from build123d import *

# Parameters (mm, degrees)
BOSS_EXTRUDE1_DEPTH      = 40
BOSS_EXTRUDE1_DEPTH_BACK = 24.13
SKETCH1_W                = 138
SKETCH1_H                = 88
SHELL1_T                 = -4
SKETCH10_W               = 12.954
SKETCH10_H               = 10.922
CUT_EXTRUDE1_DEPTH       = 4
SKETCH12_W               = 9.254
SKETCH12_H               = 11.254
CUT_EXTRUDE2_DEPTH       = 4


with BuildPart() as part:
    # Sketch1 → Boss-Extrude1 (new, two sides: drawn at the far end of the back side and taken through both)
    with BuildSketch(Plane(origin=(0, 0, 0), x_dir=(1, 0, 0), z_dir=(0, 1, 0)).offset(-BOSS_EXTRUDE1_DEPTH_BACK)):
        with Locations((29.3125, -12.885)):
            Rectangle(SKETCH1_W, SKETCH1_H)
    extrude(amount=BOSS_EXTRUDE1_DEPTH + BOSS_EXTRUDE1_DEPTH_BACK)

    # Shell1
    shell1_openings = [part.faces().sort_by_distance(p)[0] for p in [
        (29.3125, 40, 12.885),
    ]]
    offset(amount=SHELL1_T, openings=shell1_openings, kind=Kind.INTERSECTION)

    # Sketch10 → Cut-Extrude1 (cut)
    with BuildSketch(Plane.ZY.offset(-98.3125)):
        with Locations((-10.795, -11.176)):
            Rectangle(SKETCH10_W, SKETCH10_H)
    extrude(amount=CUT_EXTRUDE1_DEPTH, mode=Mode.SUBTRACT)

    # Sketch12 → Cut-Extrude2 (cut)
    with BuildSketch(Plane.ZY.offset(-98.3125)):
        with Locations((18.36, -11.01)):
            Rectangle(SKETCH12_W, SKETCH12_H)
    extrude(amount=CUT_EXTRUDE2_DEPTH, mode=Mode.SUBTRACT)


solid = part.part
The listing builds one solid part. Answer for the finished solid, in the listing's coordinates (mm). A direction names the side the tool comes from. Round coordinates to 2 decimals unless told otherwise and drop trailing zeros. Order: outer loops, then holes, each group sorted by start corner. A loop starts at its lowest first (then second) coordinate and runs counter-clockwise, first axis right, second up. Notation, with made-up numbers: (89.25, -1) - (100.25, -1) arc R21 cw to (100.25, 9) - close; hole circle Ø6 at (88, 8). An arc over 180 degrees is marked (long way). Write item = value, one per line. Start each with the question number.
1) Straight lines are drawn through the part: L1, parallel to X at y = 34.5, z = 5; L2, parallel to Z at x = 3.5, y = -12.5 (3 decimals); L3, parallel to Y at x = 90.5, z = -8.5. For each, find the intervals that lie inside material, in ascending order.
2) Section A-A, the plane z = 19 is taken. Write down the section's boundary in (x, y), plus the area to 3 significant figures.
3) Given pin 1 (10 mm diameter, centred on x = 84, z = -14, fed in from +Y), flat-ended and moving along its own axis, determine where the tip first touches the part or whether it passes through.
4) For faces 4 (the flat face through (98.312, 7, 14)), 5 (the flat face through (96, -11, 22.987)), 6 (the flat face through (28, 10, -27.115)), determine the directions among +Z, -Z, +X, -X, +Y, -Y from which every point of the face is accessible in a straight line to the end or side of a thin tool.
5) For a pull along Z with two mould halves and no side action, classify faces 1 (the flat face through (28, 7, -31.115)), 2 (the flat face through (-39.688, 7, 14)), 3 (the flat face through (94.312, 10, 13)) as released by +Z, released by -Z, zero draft, split by the parting line, or undercut.
6) Section D-D, the plane x = 33 is taken. Write down the section's boundary in (y, z) (3 decimals), plus the area to 3 significant figures.
7) Section C-C, the plane y = 23.5 is taken. Write down the section's boundary in (x, z) (1 decimal), plus the area to 3 significant figures.
8) Section B-B, the plane y = -14.5 is taken. Write down the section's boundary in (x, z) (1 decimal), plus the area to 3 significant figures.
Results list:
q1.L1 = -39.69 to -35.69, 94.31 to 98.31
q1.L2 = -31.115 to -27.115, 52.885 to 56.885
q1.L3 = -24.13 to -20.13
q2.outline = (-39.69, -24.13) - (98.31, -24.13) - (98.31, -16.64) - (94.31, -16.64) - (94.31, -20.13) - (-35.69, -20.13) - (-35.69, 40) - (-39.69, 40) - close; (94.31, -5.38) - (98.31, -5.38) - (98.31, 40) - (94.31, 40) - close
q2.area = 988 mm^2
q3.pin_1 = -20.13
q4.face_4 = +Z, -Z, +X, +Y, -Y
q4.face_5 = +X
q4.face_6 = +Y
q5.face_1 = released by -Z
q5.face_2 = zero draft
q5.face_3 = undercut
q6.outline = (-24.13, -31.115) - (40, -31.115) - (40, -27.115) - (-20.13, -27.115) - (-20.13, 52.885) - (40, 52.885) - (40, 56.885) - (-24.13, 56.885) - close
q6.area = 833 mm^2
q7.outline = (-39.7, -31.1) - (98.3, -31.1) - (98.3, 56.9) - (-39.7, 56.9) - close; hole (-35.7, -27.1) - (94.3, -27.1) - (94.3, 52.9) - (-35.7, 52.9) - close
q7.area = 1,740 mm^2
q8.outline = (-39.7, -31.1) - (98.3, -31.1) - (98.3, -17.3) - (94.3, -17.3) - (94.3, -27.1) - (-35.7, -27.1) - (-35.7, 52.9) - (94.3, 52.9) - (94.3, 23) - (98.3, 23) - (98.3, 56.9) - (-39.7, 56.9) - close; (94.3, -4.3) - (98.3, -4.3) - (98.3, 13.7) - (94.3, 13.7) - close
q8.area = 1,660 mm^2
